```python
from build123d import *

# Parameters (mm, degrees)
SKETCH1_W           = 25.6
SKETCH1_H           = 5.8
BOSS_EXTRUDE1_DEPTH = 3
SKETCH1_4_R         = 2.9
BOSS_EXTRUDE2_DEPTH = 4


with BuildPart() as part:
    # Sketch1 → Boss-Extrude1 (new body)
    with BuildSketch(Plane(origin=(0, 0, 0), x_dir=(1, 0, 0), z_dir=(0, 1, 0))):
        with Locations((12.8, 2.9)):
            Rectangle(SKETCH1_W, SKETCH1_H)
    extrude(amount=-BOSS_EXTRUDE1_DEPTH)

    # Sketch1_4 → Boss-Extrude2 (add)
    with BuildSketch(Plane(origin=(0, 0, 0), x_dir=(1, 0, 0), z_dir=(0, 1, 0))):
        with Locations(Location((2.9, 2.9, 0), (0, 0, 270))):
            Circle(SKETCH1_4_R)
        with BuildLine():
            ThreePointArc((12.8, 5.8), (9.9, 2.9), (12.8, 0))
            Line((12.8, 0), (12.8, 5.8))
        make_face()
        with BuildLine():
            Line((13.7, 5.8), (12.8, 5.8))
            ThreePointArc((12.8, 5.8), (13.255659809, 5.763978725), (13.7, 5.65680975))
            Line((13.7, 5.65680975), (13.7, 5.8))
        make_face()
        with BuildLine():
            ThreePointArc((13.7, 0.14319025), (13.255659809, 0.036021275), (12.8, 0))
            Line((12.8, 0), (13.7, 0))
            Line((13.7, 0), (13.7, 0.14319025))
        make_face()
        with BuildLine():
            Line((12.8, 5.8), (12.8, 0))
            ThreePointArc((12.8, 0), (13.255659809, 0.036021275), (13.7, 0.14319025))
            Line((13.7, 0.14319025), (13.7, 5.65680975))
            ThreePointArc((13.7, 5.65680975), (13.255659809, 5.763978725), (12.8, 5.8))
        make_face()
        with BuildLine():
            ThreePointArc((22.7, 5.8), (19.8, 2.9), (22.7, 0))
            Line((22.7, 0), (22.7, 5.8))
        make_face()
        with BuildLine():
            Line((22.7, 5.8), (22.7, 0))
            ThreePointArc((22.7, 0), (24.750609665, 0.849390335), (25.6, 2.9))
            ThreePointArc((25.6, 2.9), (24.750609665, 4.950609665), (22.7, 5.8))
        make_face()
        with BuildLine():
            Line((17.8, 5.8), (17.8, 0))
            Line((17.8, 0), (22.7, 0))
            ThreePointArc((22.7, 0), (19.8, 2.9), (22.7, 5.8))
            Line((22.7, 5.8), (17.8, 5.8))
        make_face()
    extrude(amount=BOSS_EXTRUDE2_DEPTH)


solid = part.part
```
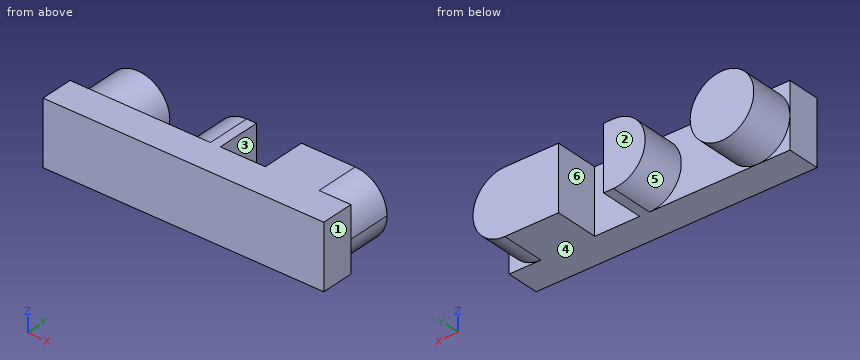
Input: part model. Units: mm. Frame: model coordinates. Face numbers are marked on the shaded views. A direction names the side the tool comes from. Coordinates: 2 decimals unless noted, no trailing zeros. Loops run counter-clockwise (first coordinate to the right, second up) from the corner with the lowest first, then second, coordinate; pieces in that order, holes last.
Q1. Mould query, pull axis X, two halves, no side actions, for the marked faces 1, 2 and 3. Classes: +X half, -X half, draft (parallel to the pull), parting line (faces both ways), or undercut.
Results are:
face 1: +X half
face 2: draft
face 3: undercut
Q2. Section D-D, the plane z = -4.05. Return the cut outline in (x, y), and give its area (3 significant figures).
Results are:
outline: (0, -3) - (25.6, -3) - (25.6, 0) - (25.36, 0) - (25.36, 4) - (17.8, 4) - (17.8, 0) - (13.7, 0) - (13.7, 4) - (10.14, 4) - (10.14, 0) - (5.56, 0) - (5.56, 4) - (0.24, 4) - (0.24, 0) - (0, 0) - close
area: 143 mm2
Q3. Section C-C, the plane x = 10.5. Return the cut outline in (y, z), and give its area (3 significant figures).
Results are:
outline: (-3, -5.8) - (0, -5.8) - (0, -4.67) - (4, -4.67) - (4, -1.13) - (0, -1.13) - (0, 0) - (-3, 0) - close
area: 31.5 mm2
Q4. Line query: line 1 along X through (y, z) = (2, -2.75); line 2 along X through (y, z) = (1, -4.7); line 3 along Y through (x, z) = (14.5, -3.3). Output: solid intervals per line, ascending.
Results are:
line 1: x = 0 to 5.8, 9.9 to 13.7, 17.8 to 25.6
line 2: x = 0.63 to 5.17, 10.53 to 13.7, 17.8 to 24.97
line 3: y = -3 to 0
Q5. Contact query for a flat-ended pin moving along its axis: pin 1 (2 mm diameter, centred on y = 3, z = -2.5, fed in from -X). Output: stop coordinate, or through.
Results are:
pin 1: stops at x = 0
Q6. Set-up query: the marked faces 4, 5 and 6. Return all of +Z, -Z, +X, -X, +Y, -Y with unobstructed straight access to the full face (end or side cutting, diameter ignored); none if empty.
Results are:
face 4: -Z, +X, -X, +Y, -Y
face 5: +Y
face 6: +Z, -Z, +Y
Q7. Section A-A, the plane y = 1.25. Return the cut outline in (x, z), and give its area (3 significant figures).
Results are:
outline: circle Ø5.8 at (2.9, -2.9); (12.8, -5.8) - (13.7, -5.8) - (13.7, 0) - (12.8, 0) arc R2.9 ccw to start; (17.8, -5.8) - (22.7, -5.8) arc R2.9 ccw to (22.7, 0) - (17.8, 0) - close
area: 86.5 mm2
